Geometry check sheet. Reference: the model listing, model coordinates, mm. A direction names the side the tool comes from. Coordinates: 2 decimals unless noted, no trailing zeros. Use CSV: the item, a comma, the result in double quotes. Start each with the question number.
```python
from build123d import *

# Parameters (mm, degrees)
SKETCH1_W           = 330
SKETCH1_H           = 330
BOSS_EXTRUDE1_DEPTH = 200
BOSS_EXTRUDE1_TAPER = 15
SKETCH2_R           = 50
CUT_EXTRUDE1_DEPTH  = 170
SKETCH7_W           = 109.8
SKETCH7_H           = 120
CUT_EXTRUDE2_DEPTH  = 50


with BuildPart() as part:
    # Sketch1 → Boss-Extrude1 (new body)
    with BuildSketch(Plane(origin=(0, 0, 0), x_dir=(1, 0, 0), z_dir=(0, 1, 0))):
        Rectangle(SKETCH1_W, SKETCH1_H)
    extrude(amount=BOSS_EXTRUDE1_DEPTH, taper=BOSS_EXTRUDE1_TAPER)

    # Sketch2 → Cut-Extrude1 (cut)
    with BuildSketch(Plane(origin=(0, 200, 0), x_dir=(1, 0, 0), z_dir=(0, 1, 0))):
        with Locations(Location((0, 0, 0), (0, 0, 270))):
            Circle(SKETCH2_R)
    extrude(amount=-CUT_EXTRUDE1_DEPTH, mode=Mode.SUBTRACT)

    # Sketch7 → Cut-Extrude2 (cut)
    with BuildSketch(Plane(origin=(0, 41.25, 153.947095812), x_dir=(1, 0, 0), z_dir=(0, 0.2588190451025208, 0.9659258262890682))):
        with Locations((0, 104.35009364)):
            Rectangle(SKETCH7_W, SKETCH7_H)
    extrude(amount=-CUT_EXTRUDE2_DEPTH, mode=Mode.SUBTRACT)


solid = part.part
```
1) Material ranges on line 1 along Z through (x, y) = (39.5, 161); line 2 along Y through (x, z) = (-20, 37.5); line 3 along X through (y, z) = (125, -1), recorded low to high.
2) Gauge pin test, flat ends, axial feed: P1, Ø1, axis at y = 174.5, z = 35, coming from the -X side; P2, Ø2, axis at y = 26.5, z = -48.5, coming from the +X side; P3, Ø8, axis at x = 11.5, y = 97, coming from the -Z side. Record the tip position at first contact, or that the pin passes through.
3) Set-up check for faces 5 (the face through (-0.77, 77.71, 118.66)), 6 (the face through (-53, 200, 0)): record each of +Z, -Z, +X, -X, +Y, -Y from which the full face is reachable in a straight line by a thin tool's end or side.
4) Draft check along Z on faces 1 (the face through (-5, 0, 0)), 2 (the face through (-0.77, 193.62, 87.6)), 3 (the face through (15.02, 116.19, 47.69)), 4 (the face through (1, 30, -1)). Enter one of: +Z half, -Z half, draft (parallel to the pull), parting line (faces both ways), or undercut.
Results are:
1,line 1,"z = -121.86 to -30.66, 30.66 to 70.1"
1,line 2,"y = 0 to 30"
1,line 3,"x = -131.51 to -49.99, 49.99 to 131.51"
2,P1,"stops at x = -118.38"
2,P2,"stops at x = 158.17"
2,P3,"stops at z = -140.08"
3,face 5,"none"
3,face 6,"+Z, -Z, +X, -X, +Y"
4,face 1,"draft"
4,face 2,"+Z half"
4,face 3,"undercut"
4,face 4,"undercut"
